Work out the finished part from the listing and answer in its coordinate system (mm). Round coordinates to 2 decimals unless told otherwise and drop trailing zeros. Write each loop counter-clockwise with the first axis right and the second up, starting at its lowest first coordinate (ties: lowest second). Pieces come first, ordered by that corner, then holes. Notation, with made-up numbers: (53.5, 75) -> (96.5, 75) arc R22 cw to (96.5, 104) -> close; hole circle Ø4 at (-6, 75.5). An arc over 180 degrees is marked (long way). One line per item, written item: value.
```python
from build123d import *

# Parameters (mm, degrees)
SKETCH1_W           = 203.2
SKETCH1_H           = 203.2
SKETCH1_W_2         = 115
SKETCH1_H_2         = 115
SKETCH1_R           = 2.25
BOSS_EXTRUDE1_DEPTH = 10
SKETCH4_R           = 3.38
CUT_EXTRUDE1_DEPTH  = 11


with BuildPart() as part:
    # Sketch1 → Boss-Extrude1 (new body)
    with BuildSketch(Plane(origin=(0, 0, 0), x_dir=(1, 0, 0), z_dir=(0, 1, 0))):
        with Locations((101.6, 101.6)):
            Rectangle(SKETCH1_W, SKETCH1_H)
        with Locations((101.6, 101.6)):
            Rectangle(SKETCH1_W_2, SKETCH1_H_2, mode=Mode.SUBTRACT)
        with Locations((101.6, 101.6)):
            Rectangle(SKETCH1_W_2, SKETCH1_H_2)
        with Locations((51.6, 151.6)):
            Circle(SKETCH1_R, mode=Mode.SUBTRACT)
        with Locations((151.6, 151.6)):
            Circle(SKETCH1_R, mode=Mode.SUBTRACT)
        with Locations((151.6, 51.6)):
            Circle(SKETCH1_R, mode=Mode.SUBTRACT)
        with Locations((51.6, 51.6)):
            Circle(SKETCH1_R, mode=Mode.SUBTRACT)
    extrude(amount=BOSS_EXTRUDE1_DEPTH)

    # Sketch4 → Cut-Extrude1 (cut, through all)
    with BuildSketch(Plane(origin=(0, 10, 0), x_dir=(1, 0, 0), z_dir=(0, 1, 0))):
        with Locations((12.7, 101.6)):
            Circle(SKETCH4_R)
        with Locations((190.5, 101.6)):
            Circle(SKETCH4_R)
        with Locations((101.6, 190.5)):
            Circle(SKETCH4_R)
        with Locations((101.6, 12.7)):
            Circle(SKETCH4_R)
    extrude(amount=-CUT_EXTRUDE1_DEPTH, mode=Mode.SUBTRACT)


solid = part.part
```
(1) Find section B-B on z = -101.6. Give the vertices of the cut face in (x, y), plus the area to 3 significant figures.
Reported:
outline: (0, 0) -> (9.32, 0) -> (9.32, 10) -> (0, 10) -> close; (16.08, 0) -> (187.12, 0) -> (187.12, 10) -> (16.08, 10) -> close; (193.88, 0) -> (203.2, 0) -> (203.2, 10) -> (193.88, 10) -> close
area: 1,900 mm2
(2) Find section D-D on x = 190.5. Give the vertices of the cut face in (y, z).
Reported:
outline: (0, -203.2) -> (10, -203.2) -> (10, -104.98) -> (0, -104.98) -> close; (0, -98.22) -> (10, -98.22) -> (10, 0) -> (0, 0) -> close
(3) Consider probe 1 along Z at (x, y) = (151.6, 6.5); probe 2 along X at (y, z) = (7.5, -151.6); probe 3 along X at (y, z) = (3, -190.5). Determine where each line is inside the solid, lowest interval first.
Reported:
probe 1: z = -203.2 to -153.85, -149.35 to -53.85, -49.35 to 0
probe 2: x = 0 to 49.35, 53.85 to 149.35, 153.85 to 203.2
probe 3: x = 0 to 98.22, 104.98 to 203.2
(4) Find section A-A on z = -12.7. Give the vertices of the cut face in (x, y).
Reported:
outline: (0, 0) -> (98.22, 0) -> (98.22, 10) -> (0, 10) -> close; (104.98, 0) -> (203.2, 0) -> (203.2, 10) -> (104.98, 10) -> close
(5) A flat-ended cylindrical pin translates along its axis: pin 1 Ø6 at (x, z) = (101.6, -190.5) entering from -Y. Find the tip coordinate at first contact, or state that the pin passes through.
Reported:
pin 1: passes through
(6) For a pull along Z with two mould halves and no side action, classify faces 1 (the face through (100, 5, -203.2)), 2 (the face through (103.42, 5.07, -193.35)), 3 (the face through (100, 5, 0)) as pulls with the +Z half, pulls with the -Z half, needs draft (parallel to the pull), parting line crosses it, or undercut.
Reported:
face 1: pulls with the -Z half
face 2: undercut
face 3: pulls with the +Z half
(7) Find section C-C on x = 101.6. Give the vertices of the cut face in (y, z).
Reported:
outline: (0, -203.2) -> (10, -203.2) -> (10, -193.88) -> (0, -193.88) -> close; (0, -187.12) -> (10, -187.12) -> (10, -16.08) -> (0, -16.08) -> close; (0, -9.32) -> (10, -9.32) -> (10, 0) -> (0, 0) -> close
